Work out the finished part from the listing and answer in its coordinate system (mm). A direction names the side the tool comes from. Coordinates: 2 decimals unless noted, no trailing zeros. Write each loop counter-clockwise with the first axis right and the second up, starting at its lowest first coordinate (ties: lowest second). Pieces come first, ordered by that corner, then holes. Notation, with made-up numbers: M 31,17 L 61,17 A21 ccw 61,36 Z; hole C 83.25,-6 d4. An arc over 180 degrees is marked long. Answer as CSV lines item,"result". Start each with the question number.
(1) A cutting plane is placed at C-C on x = 40.5. Give the vertices of the cut face in (y, z).
(2) For faces 1 (the flat face through (130, 64, -60.101)), 2 (the flat face through (102, 127, -5)), 3 (the flat face through (83, 84, 60.101)), determine the directions among +Z, -Z, +X, -X, +Y, -Y from which every point of the face is accessible in a straight line to the end or side of a thin tool.
(3) The mould has two halves that part along X. Classify faces 4 (the cylindrical face through (115.758, 42.694, 66.54)), 5 (the flat face through (207.425, 119, -5)), 6 (the flat face through (0, 63, -5)): released by +X, released by -X, zero draft, split by the parting line, or undercut.
(4) A cutting plane is placed at B-B on x = 102. Give the vertices of the cut face in (y, z), then the cut area to 3 significant figures.
(5) A cutting plane is placed at A-A on y = 44.5. Give the vertices of the cut face in (x, z), then the cut area to 3 significant figures.
(6) A cutting plane is placed at D-D on z = 47. Give the vertices of the cut face in (x, y), then the cut area to 3 significant figures.
(7) Find the intervals of material crossed by L1, parallel to Z at x = 183, y = 106; L2, parallel to Y at x = 22.5, z = -40.5; L3, parallel to X at y = 95, z = 28, in increasing order. Write a range as [from, to].
from build123d import *

# Parameters (mm, degrees)
F0_W     = 207.425324
F0_H     = 127
F1_DEPTH = 72.80146
F2_SIZE  = 12.7
F3_T     = -12.7
F4_R     = 25.4
F5_DEPTH = 148.94068


with BuildPart() as f1:
    # F0 (on Top) → F1 (new body, symmetric)
    with BuildSketch(Plane.XY):
        with Locations((103.712662, 63.5)):
            Rectangle(F0_W, F0_H)
    extrude(amount=F1_DEPTH, both=True)

    # F2
    f2_edges = [f1.edges().sort_by_distance(p)[0] for p in [
        (207.425324, 63.5, 72.80146),
        (103.712662, 127, 72.80146),
        (0, 63.5, 72.80146),
        (103.712662, 0, 72.80146),
    ]]
    chamfer(f2_edges, length=F2_SIZE)

    # F3
    f3_openings = [f1.faces().sort_by_distance(p)[0] for p in [
        (207.425324, 63.5, -6.35),
    ]]
    offset(amount=F3_T, openings=f3_openings)

    # F4 (on face) → F5 (cut)
    with BuildSketch(Plane.XY.offset(72.80146)):
        with Locations((104.037382, 65.22774)):
            Circle(F4_R)
    extrude(amount=-F5_DEPTH, mode=Mode.SUBTRACT)


solid = f1.part
Here are the results:
1,outline,"M 0,-72.8 L 127,-72.8 L 127,60.1 L 114.3,72.8 L 12.7,72.8 L 0,60.1 Z; hole M 12.7,-60.1 L 114.3,-60.1 L 114.3,54.84 L 109.04,60.1 L 17.96,60.1 L 12.7,54.84 Z"
2,face 1,"+X"
2,face 2,"+Z, -Z, +X, -X, +Y"
2,face 3,"none"
3,face 4,"undercut"
3,face 5,"released by +X"
3,face 6,"released by -X"
4,outline,"M 0,-72.8 L 39.91,-72.8 L 39.91,-60.1 L 12.7,-60.1 L 12.7,54.84 L 17.96,60.1 L 39.91,60.1 L 39.91,72.8 L 12.7,72.8 L 0,60.1 Z; M 90.55,-72.8 L 127,-72.8 L 127,60.1 L 114.3,72.8 L 90.55,72.8 L 90.55,60.1 L 109.04,60.1 L 114.3,54.84 L 114.3,-60.1 L 90.55,-60.1 Z"
4,area,"4,860 mm^2"
5,outline,"M 0,-72.8 L 89.36,-72.8 L 89.36,-60.1 L 12.7,-60.1 L 12.7,54.84 L 17.96,60.1 L 89.36,60.1 L 89.36,72.8 L 12.7,72.8 L 0,60.1 Z; M 118.72,-72.8 L 207.43,-72.8 L 207.43,-60.1 L 118.72,-60.1 Z; M 118.72,60.1 L 189.46,60.1 L 207.43,42.14 L 207.43,60.1 L 194.73,72.8 L 118.72,72.8 Z"
5,area,"6,060 mm^2"
6,outline,"M 0,0 L 207.43,0 L 207.43,127 L 0,127 Z; hole M 12.7,12.7 L 202.57,12.7 L 202.57,114.3 L 12.7,114.3 Z"
6,area,"7,050 mm^2"
7,L1,"z = [-72.8, -60.1], [60.1, 72.8]"
7,L2,"y = [0, 12.7], [114.3, 127]"
7,L3,"x = [0, 12.7]"
